Read the model definition and answer for the solid it produces. Units are mm, in the model's axes. Give positions to 0.01 mm unless a question says otherwise; leave off trailing zeros. Order: outer loops, then holes, each group sorted by start corner. A loop starts at its lowest first (then second) coordinate and runs counter-clockwise, first axis right, second up.
```python
from build123d import *

# Parameters (mm, degrees)
SKETCH1_R           = 40
SKETCH1_R_2         = 2.25
BOSS_EXTRUDE1_DEPTH = 3


with BuildPart() as part:
    # Sketch1 → Boss-Extrude1 (new body)
    with BuildSketch(Plane(origin=(0, 0, 0), x_dir=(1, 0, 0), z_dir=(0, 1, 0))):
        Polygon((75.462130999, 64.93515636), (-288.537869001, 64.93515636), (-288.537869001, 22.43515636), (-291.537869001, 22.43515636), (-291.537869001, 7.43515636), (-288.537869001, 7.43515636), (-288.537869001, -35.06484364), (75.462130999, -35.06484364), (75.462130999, 7.43515636), (78.462130999, 7.43515636), (78.462130999, 22.43515636), (75.462130999, 22.43515636), align=None)
        with Locations(Location((-239.737869001, 14.93515636, 0), (0, 0, 270))):
            Circle(SKETCH1_R, mode=Mode.SUBTRACT)
        with Locations(Location((-203.987869001, 50.68515636, 0), (0, 0, 270))):
            Circle(SKETCH1_R_2, mode=Mode.SUBTRACT)
        with Locations(Location((-203.987869001, -20.81484364, 0), (0, 0, 90))):
            Circle(SKETCH1_R_2, mode=Mode.SUBTRACT)
        with Locations(Location((-275.487869001, -20.81484364, 0), (0, 0, 270))):
            Circle(SKETCH1_R_2, mode=Mode.SUBTRACT)
        with Locations(Location((-275.487869001, 50.68515636, 0), (0, 0, 90))):
            Circle(SKETCH1_R_2, mode=Mode.SUBTRACT)
        with Locations(Location((-186.687869001, 50.68515636, 0), (0, 0, 90))):
            Circle(SKETCH1_R_2, mode=Mode.SUBTRACT)
        with Locations(Location((-150.937869001, 14.93515636, 0), (0, 0, 270))):
            Circle(SKETCH1_R, mode=Mode.SUBTRACT)
        with Locations(Location((-115.187869001, 50.68515636, 0), (0, 0, 270))):
            Circle(SKETCH1_R_2, mode=Mode.SUBTRACT)
        with Locations(Location((-186.687869001, -20.81484364, 0), (0, 0, 270))):
            Circle(SKETCH1_R_2, mode=Mode.SUBTRACT)
        with Locations(Location((-115.187869001, -20.81484364, 0), (0, 0, 90))):
            Circle(SKETCH1_R_2, mode=Mode.SUBTRACT)
        with Locations(Location((-97.887869001, 50.68515636, 0), (0, 0, 90))):
            Circle(SKETCH1_R_2, mode=Mode.SUBTRACT)
        with Locations(Location((-62.137869001, 14.93515636, 0), (0, 0, 270))):
            Circle(SKETCH1_R, mode=Mode.SUBTRACT)
        with Locations(Location((-26.387869001, 50.68515636, 0), (0, 0, 270))):
            Circle(SKETCH1_R_2, mode=Mode.SUBTRACT)
        with Locations(Location((-97.887869001, -20.81484364, 0), (0, 0, 270))):
            Circle(SKETCH1_R_2, mode=Mode.SUBTRACT)
        with Locations(Location((-26.387869001, -20.81484364, 0), (0, 0, 90))):
            Circle(SKETCH1_R_2, mode=Mode.SUBTRACT)
        with Locations(Location((-9.087869001, 50.68515636, 0), (0, 0, 90))):
            Circle(SKETCH1_R_2, mode=Mode.SUBTRACT)
        with Locations(Location((26.662130999, 14.93515636, 0), (0, 0, 270))):
            Circle(SKETCH1_R, mode=Mode.SUBTRACT)
        with Locations(Location((62.412130999, 50.68515636, 0), (0, 0, 270))):
            Circle(SKETCH1_R_2, mode=Mode.SUBTRACT)
        with Locations(Location((-9.087869001, -20.81484364, 0), (0, 0, 270))):
            Circle(SKETCH1_R_2, mode=Mode.SUBTRACT)
        with Locations(Location((62.412130999, -20.81484364, 0), (0, 0, 90))):
            Circle(SKETCH1_R_2, mode=Mode.SUBTRACT)
    extrude(amount=BOSS_EXTRUDE1_DEPTH)


solid = part.part
```
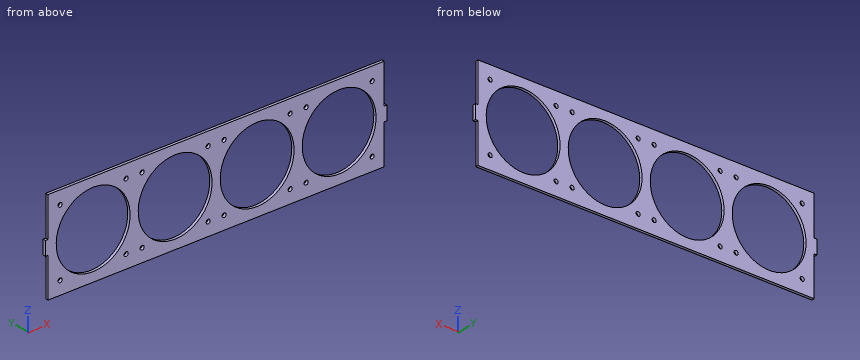
1) The part is cut by section B-B on z = 7. Determine the outline of the cut face in (x, y).
Final values:
outline: (-288.54, 0) - (-273.19, 0) - (-273.19, 3) - (-288.54, 3) - close; (-206.29, 0) - (-184.39, 0) - (-184.39, 3) - (-206.29, 3) - close; (-117.49, 0) - (-95.59, 0) - (-95.59, 3) - (-117.49, 3) - close; (-28.69, 0) - (-6.79, 0) - (-6.79, 3) - (-28.69, 3) - close; (60.11, 0) - (75.46, 0) - (75.46, 3) - (60.11, 3) - close
2) The part is cut by section D-D on x = -235.5. Determine the outline of the cut face in (y, z), and give its area (3 significant figures).
Final values:
outline: (0, -64.94) - (3, -64.94) - (3, -54.71) - (0, -54.71) - close; (0, 24.84) - (3, 24.84) - (3, 35.06) - (0, 35.06) - close
area: 61.4 mm2
3) The part is cut by section A-A on x = -155.5. Determine the outline of the cut face in (y, z).
Final values:
outline: (0, -64.94) - (3, -64.94) - (3, -54.67) - (0, -54.67) - close; (0, 24.8) - (3, 24.8) - (3, 35.06) - (0, 35.06) - close
4) Given pin 1 (12 mm diameter, centred on x = -192, z = 3.5, fed in from -Y); pin 2 (0.9 mm diameter, centred on y = 1, z = -46, fed in from -X); pin 3 (1.5 mm diameter, centred on y = 1.5, z = -34.5, fed in from +X), each flat-ended and moving along its own axis, determine where each tip first touches the part or whether it passes through.
Final values:
pin 1: stops at y = 0
pin 2: stops at x = -288.54
pin 3: stops at x = 75.46
5) Consider L1, parallel to X at y = 0.35, z = -36; L2, parallel to Z at x = -150, y = 1.3; L3, parallel to Z at x = -28, y = 1.4. Determine where each line is inside the solid, lowest interval first.
Final values:
L1: x = -288.54 to -273.74, -205.73 to -184.94, -116.93 to -96.14, -28.13 to -7.34, 60.67 to 75.46
L2: z = -64.94 to -54.92, 25.05 to 35.06
L3: z = -64.94 to -52.25, -49.12 to -35.78, 5.91 to 19.25, 22.38 to 35.06
6) The part is cut by section C-C on y = 2. Count the separate pieces of the cut face and the enclosed holes in it, and give its area (3 significant figures).
Final values:
separate pieces: 1
enclosed holes: 20
area: 16,100 mm2
